Read the model definition and answer for the solid it produces. Units are mm, in the model's axes. A direction names the side the tool comes from. Coordinates: 2 decimals unless noted, no trailing zeros. Order: outer loops, then holes, each group sorted by start corner. A loop starts at its lowest first (then second) coordinate and runs counter-clockwise, first axis right, second up. Notation, with made-up numbers: (1, -39.5) - (21, -39.5) arc R11 cw to (21, -32.5) - close; hole circle Ø11 at (5, 74). An arc over 180 degrees is marked (long way). Use one line per item in the form item = value.
```python
from build123d import *

# Parameters (mm, degrees)
SKETCH_1_W          = 55
SKETCH_1_H          = 30
SKETCH_1_R          = 1.65
EXTRUDE_1_DEPTH     = 3
SKETCH_2_W          = 55
SKETCH_2_H          = 30
EXTRUDE_2_DEPTH     = 3
EXTRUDE_3_DEPTH     = 3
SKETCH_8_R          = 1.65
CUT_EXTRUDE_1_DEPTH = 10
FILLET_1_R          = 5
FILLET_2_R          = 3
CUT_EXTRUDE_2_DEPTH = 10
CUT_EXTRUDE_3_DEPTH = 4
CUT_EXTRUDE_4_DEPTH = 4
FILLET_3_R          = 2


with BuildPart() as part:
    # 草图1 → 凸台-拉伸1 (new body)
    with BuildSketch(Plane.XY):
        with Locations((0, 11.5)):
            Rectangle(SKETCH_1_W, SKETCH_1_H)
        with Locations((-22.5, 0)):
            Circle(SKETCH_1_R, mode=Mode.SUBTRACT)
        with Locations((-22.5, 22)):
            Circle(SKETCH_1_R, mode=Mode.SUBTRACT)
        with Locations((22.5, 22)):
            Circle(SKETCH_1_R, mode=Mode.SUBTRACT)
        with Locations((22.5, 0)):
            Circle(SKETCH_1_R, mode=Mode.SUBTRACT)
    extrude(amount=EXTRUDE_1_DEPTH)

    # 草图2 → 凸台-拉伸2 (add)
    with BuildSketch(Plane.XY.offset(3)):
        with Locations((0, 41.5)):
            Rectangle(SKETCH_2_W, SKETCH_2_H)
    extrude(amount=-EXTRUDE_2_DEPTH)

    # 草图4 → 凸台-拉伸3 (add)
    with BuildSketch(Plane.XY.offset(3)):
        Polygon((-27.5, 26.5), (-72.5, 26.5), (-42.5, 56.5), (-27.5, 56.5), align=None)
    extrude(amount=-EXTRUDE_3_DEPTH)

    # 草图8 → 切除-拉伸1 (cut)
    with BuildSketch(Plane(origin=(0, 0, 0), x_dir=(-1, 0, 0), z_dir=(0, 0, -1))):
        with Locations((50.378679656, 44.378679656)):
            Circle(SKETCH_8_R)
    extrude(amount=-CUT_EXTRUDE_1_DEPTH, mode=Mode.SUBTRACT)

    # 圆角1
    fillet_1_edges = [part.edges().sort_by_distance(p)[0] for p in [
        (-27.5, 26.5, 1.5),
    ]]
    fillet(fillet_1_edges, radius=FILLET_1_R)

    # 圆角2
    fillet_2_edges = [part.edges().sort_by_distance(p)[0] for p in [
        (27.5, 56.5, 1.5),
        (-42.5, 56.5, 1.5),
        (-72.5, 26.5, 1.5),
        (27.5, -3.5, 1.5),
        (-27.5, -3.5, 1.5),
    ]]
    fillet(fillet_2_edges, radius=FILLET_2_R)

    # 草图9 → 切除-拉伸2 (cut)
    with BuildSketch(Plane(origin=(0, 0, 0), x_dir=(-1, 0, 0), z_dir=(0, 0, -1))):
        with BuildLine():
            Line((17.5, 53), (27.5, 53))
            ThreePointArc((27.5, 53), (29, 51.5), (27.5, 50))
            Line((27.5, 50), (17.5, 50))
            ThreePointArc((17.5, 50), (16, 51.5), (17.5, 53))
        make_face()
    extrude(amount=-CUT_EXTRUDE_2_DEPTH, mode=Mode.SUBTRACT)

    # 草图10 → 切除-拉伸3 (cut, through all)
    with BuildSketch(Plane(origin=(0, 0, 0), x_dir=(-1, 0, 0), z_dir=(0, 0, -1))):
        with BuildLine():
            Line((-15.5, 6.5), (15.5, 6.5))
            ThreePointArc((15.5, 6.5), (16.914213562, 7.085786438), (17.5, 8.5))
            Line((17.5, 8.5), (17.5, 21.5))
            ThreePointArc((17.5, 21.5), (21.893398282, 32.106601718), (32.5, 36.5))
            Line((32.5, 36.5), (43.529437252, 36.5))
            ThreePointArc((43.529437252, 36.5), (45.377196317, 37.734633135), (44.943650814, 39.914213562))
            Line((44.943650814, 39.914213562), (38.943650814, 45.914213562))
            ThreePointArc((38.943650814, 45.914213562), (38.294804116, 46.347759065), (37.529437252, 46.5))
            Line((37.529437252, 46.5), (-15.5, 46.5))
            ThreePointArc((-15.5, 46.5), (-16.914213562, 45.914213562), (-17.5, 44.5))
            Line((-17.5, 44.5), (-17.5, 8.5))
            ThreePointArc((-17.5, 8.5), (-16.914213562, 7.085786438), (-15.5, 6.5))
        make_face()
    extrude(amount=-CUT_EXTRUDE_3_DEPTH, mode=Mode.SUBTRACT)

    # 草图11 → 切除-拉伸4 (cut, through all)
    with BuildSketch(Plane(origin=(0, 0, 0), x_dir=(-1, 0, 0), z_dir=(0, 0, -1))):
        with BuildLine():
            Line((-27.5, 24.5), (12.5, 24.5))
            Line((12.5, 24.5), (12.5, 56.5))
            Line((12.5, 56.5), (-24.5, 56.5))
            ThreePointArc((-24.5, 56.5), (-26.621320344, 55.621320344), (-27.5, 53.5))
            Line((-27.5, 53.5), (-27.5, 24.5))
        make_face()
    extrude(amount=-CUT_EXTRUDE_4_DEPTH, mode=Mode.SUBTRACT)

    # 圆角3
    fillet_3_edges = [part.edges().sort_by_distance(p)[0] for p in [
        (-12.5, 46.5, 1.5),
        (17.5, 24.5, 1.5),
        (-12.5, 56.5, 1.5),
        (27.5, 24.5, 1.5),
    ]]
    fillet(fillet_3_edges, radius=FILLET_3_R)


solid = part.part
```
(1) Given pin 1 Ø1.5 at (x, z) = (-7.5, 1.5) entering from +Y; pin 2 Ø1.5 at (x, z) = (22, 1.5) entering from +Y; pin 3 Ø1.5 at (y, z) = (12.5, 2) entering from -X, each flat-ended and moving along its own axis, determine where each tip first touches the part or whether it passes through.
Answer list:
pin_1 = 6.5
pin_2 = 24.5
pin_3 = -27.5
(2) Section B-B, the plane x = 22.5 is taken. Write down the section's boundary in (y, z).
Answer list:
outline = (-3.5, 0) - (-1.65, 0) - (-1.65, 3) - (-3.5, 3) - close; (1.65, 0) - (20.35, 0) - (20.35, 3) - (1.65, 3) - close; (23.65, 0) - (24.5, 0) - (24.5, 3) - (23.65, 3) - close
(3) Section C-C, the plane x = -30.5 is taken. Write down the section's boundary in (y, z).
Answer list:
outline = (26.08, 0) - (36.37, 0) - (36.37, 3) - (26.08, 3) - close; (46.5, 0) - (56.5, 0) - (56.5, 3) - (46.5, 3) - close
(4) Section A-A, the plane y = 51.5 is taken. Write down the section's boundary in (x, z), then the cut area to 3 significant figures.
Answer list:
outline = (-47.5, 0) - (-29, 0) - (-29, 3) - (-47.5, 3) - close; (-16, 0) - (-12.5, 0) - (-12.5, 3) - (-16, 3) - close
area = 66.0 mm2
(5) Which of the six approach directions +Z, -Z, +X, -X, +Y, -Y give full straight-line access (tool end or side, diameter ignored) to faces 1 (the cylindrical face through (16.93, 7.1, 1.48)), 2 (the cylindrical face through (-16, 51.5, 1.5)), 3 (the flat face through (-27.5, 10, 2))?
Answer list:
face_1 = +Z, -Z, +Y
face_2 = +Z, -Z
face_3 = +Z, -Z, -X, -Y
(6) Section D-D, the plane z = 1.9 is taken. State how many separate pieces and enclosed holes the cut face has, then the cut area to 3 significant figures.
Answer list:
separate_pieces = 1
enclosed_holes = 6
area = 1,790 mm2
(7) The mould has two halves that part along X. Classify faces 4 (the cylindrical face through (-29, 25.07, 1.48)), 5 (the cylindrical face through (26.93, 23.9, 1.52)), 6 (the cylindrical face through (20.85, 0.07, 1.48)): +X half, -X half, draft (parallel to the pull), parting line (faces both ways), or undercut.
Answer list:
face_4 = -X half
face_5 = +X half
face_6 = undercut
(8) Straight lines are drawn through the part: L1, parallel to Y at x = 22.5, z = 2.4; L2, parallel to Y at x = 24, z = 0.7; L3, parallel to Y at x = -33, z = 2. For each, find the intervals that lie inside material, in ascending order.
Answer list:
L1 = -3.5 to -1.65, 1.65 to 20.35, 23.65 to 24.5
L2 = -3.5 to -0.69, 0.69 to 21.31, 22.69 to 24.5
L3 = 26.5 to 36.5, 46.5 to 56.5
